Design review of the part built by this model. Coordinates are the model's own, in mm. Face numbers are marked on the shaded views. A direction names the side the tool comes from. Coordinates: 2 decimals unless noted, no trailing zeros. Order: outer loops, then holes, each group sorted by start corner. A loop starts at its lowest first (then second) coordinate and runs counter-clockwise, first axis right, second up. Notation, with made-up numbers: (61, 83.5) -> (110, 83.5) arc R26 cw to (110, 97.5) -> close; hole circle Ø11 at (52.5, 71.25). An arc over 180 degrees is marked (long way). Write item = value, one per line.
```python
from build123d import *

# Parameters (mm, degrees)
SKETCH1_W                    = 160
SKETCH1_H                    = 120
BOSS_EXTRUDE1_DEPTH          = 70
CUT_EXTRUDE1_DEPTH           = 70
M20_TAPPED_HOLE3_D           = 17.5
M20_TAPPED_HOLE3_DEPTH       = 30
M20_TAPPED_HOLE3_CBORE_D     = 20
M20_TAPPED_HOLE3_CBORE_DEPTH = 25
M20_TAPPED_HOLE3_TIP         = 5.257530416
F_20_0MM_DOWEL_SLOT1_D       = 20
F_20_0MM_DOWEL_SLOT1_DEPTH   = 40
F_20_0MM_DOWEL_SLOT1_TIP     = 6.00860619
SKETCH16_R                   = 10
CUT_EXTRUDE3_DEPTH           = 40
CUT_EXTRUDE4_DEPTH           = 40
SKETCH18_R                   = 10
BOSS_EXTRUDE2_DEPTH          = 40
CUT_EXTRUDE6_DEPTH           = 20
SKETCH20_R                   = 10
CUT_EXTRUDE7_DEPTH           = 71
SKETCH21_R                   = 10
CUT_EXTRUDE8_DEPTH           = 20
CUT_EXTRUDE11_DEPTH          = 20
CUT_EXTRUDE12_DEPTH          = 20
SKETCH25_R                   = 20
SKETCH25_R_2                 = 10
BOSS_EXTRUDE6_DEPTH          = 10
RIB1_REACH                   = 186.662
SKETCH26_WALL_W              = 391.050063724
SKETCH26_WALL_H              = 10


with BuildPart() as part:
    # Sketch1 → Boss-Extrude1 (new body)
    with BuildSketch(Plane.XY):
        with Locations((80, 60)):
            Rectangle(SKETCH1_W, SKETCH1_H)
    extrude(amount=BOSS_EXTRUDE1_DEPTH)

    # Sketch2 → Cut-Extrude1 (cut)
    with BuildSketch(Plane.XY.offset(70)):
        with BuildLine():
            Line((60, 120), (0, 120))
            Line((0, 120), (0, 60))
            ThreePointArc((0, 60), (17.573593129, 102.426406871), (60, 120))
        make_face()
        with BuildLine():
            ThreePointArc((60, 0), (17.573593129, 17.573593129), (0, 60))
            Line((0, 60), (0, 0))
            Line((0, 0), (60, 0))
        make_face()
    extrude(amount=-CUT_EXTRUDE1_DEPTH, mode=Mode.SUBTRACT)

    # M20 Tapped Hole3
    with Locations(Plane(origin=(140, 100, 70), x_dir=(1, 0, 0), z_dir=(0, 0, 1))):
        with Locations((0, 0), (0, -80)):
            CounterBoreHole(M20_TAPPED_HOLE3_D / 2, M20_TAPPED_HOLE3_CBORE_D / 2, M20_TAPPED_HOLE3_CBORE_DEPTH, depth=M20_TAPPED_HOLE3_DEPTH)
            with Locations((0, 0, -(M20_TAPPED_HOLE3_DEPTH + M20_TAPPED_HOLE3_TIP / 2))):  # 118° drill point
                Cone(0, M20_TAPPED_HOLE3_D / 2, M20_TAPPED_HOLE3_TIP, mode=Mode.SUBTRACT)

    # 20.0mm Dowel Slot1
    with Locations(Plane.XY.offset(70)):
        with Locations((60, 60)):
            Hole(F_20_0MM_DOWEL_SLOT1_D / 2, depth=F_20_0MM_DOWEL_SLOT1_DEPTH)
            with Locations((0, 0, -(F_20_0MM_DOWEL_SLOT1_DEPTH + F_20_0MM_DOWEL_SLOT1_TIP / 2))):  # 118° drill point
                Cone(0, F_20_0MM_DOWEL_SLOT1_D / 2, F_20_0MM_DOWEL_SLOT1_TIP, mode=Mode.SUBTRACT)

    # Sketch16 → Cut-Extrude3 (cut)
    with BuildSketch(Plane.XY.offset(70)):
        with BuildLine():
            ThreePointArc((28.775010008, 35), (100, 60), (28.775010008, 85))
            Line((28.775010008, 85), (5.456439427, 85))
            ThreePointArc((5.456439427, 85), (0, 60), (5.456439427, 35))
            Line((5.456439427, 35), (28.775010008, 35))
        make_face()
        with Locations((60, 60)):
            Circle(SKETCH16_R, mode=Mode.SUBTRACT)
    extrude(amount=-CUT_EXTRUDE3_DEPTH, mode=Mode.SUBTRACT)

    # Sketch17 → Cut-Extrude4 (cut)
    with BuildSketch(Plane.XY.offset(30)):
        with BuildLine():
            Line((5.456439427, 85), (28.775010008, 85))
            ThreePointArc((28.775010008, 85), (42.679491924, 96.055512755), (60, 100))
            Line((60, 100), (15.27864045, 100))
            ThreePointArc((15.27864045, 100), (9.804072956, 92.868965731), (5.456439427, 85))
        make_face()
        with BuildLine():
            Line((28.775010008, 35), (5.456439427, 35))
            ThreePointArc((5.456439427, 35), (9.804072956, 27.131034269), (15.27864045, 20))
            Line((15.27864045, 20), (60, 20))
            ThreePointArc((60, 20), (42.679491924, 23.944487245), (28.775010008, 35))
        make_face()
    extrude(amount=CUT_EXTRUDE4_DEPTH, mode=Mode.SUBTRACT)

    # Sketch18 → Boss-Extrude2 (add)
    with BuildSketch(Plane.XY.offset(30)):
        with BuildLine():
            Line((60, 20), (15.27864045, 20))
            ThreePointArc((15.27864045, 20), (0, 60), (15.27864045, 100))
            Line((15.27864045, 100), (60, 100))
            ThreePointArc((60, 100), (100, 60), (60, 20))
        make_face()
        with Locations((60, 60)):
            Circle(SKETCH18_R, mode=Mode.SUBTRACT)
    extrude(amount=BOSS_EXTRUDE2_DEPTH)

    # Sketch19 → Cut-Extrude6 (cut)
    with BuildSketch(Plane(origin=(0, 0, 0), x_dir=(-1, 0, 0), z_dir=(0, 0, -1))):
        with BuildLine():
            ThreePointArc((-60, 99.05124838), (-43.43620227, 95.364397418), (-30, 85))
            Line((-30, 85), (-5.456439427, 85))
            ThreePointArc((-5.456439427, 85), (-9.461419592, 92.339633429), (-14.447832104, 99.05124838))
            Line((-14.447832104, 99.05124838), (-60, 99.05124838))
        make_face()
        with BuildLine():
            Line((-5.456439427, 85), (-30, 85))
            ThreePointArc((-30, 85), (-43.43620227, 95.364397418), (-60, 99.05124838))
            ThreePointArc((-60, 99.05124838), (-99.05124838, 60), (-60, 20.94875162))
            ThreePointArc((-60, 20.94875162), (-43.43620227, 24.635602582), (-30, 35))
            Line((-30, 35), (-5.456439427, 35))
            ThreePointArc((-5.456439427, 35), (0, 60), (-5.456439427, 85))
        make_face()
        with BuildLine():
            ThreePointArc((-14.447832104, 20.94875162), (-9.461419592, 27.660366571), (-5.456439427, 35))
            Line((-5.456439427, 35), (-30, 35))
            ThreePointArc((-30, 35), (-43.43620227, 24.635602582), (-60, 20.94875162))
            Line((-60, 20.94875162), (-14.447832104, 20.94875162))
        make_face()
    extrude(amount=-CUT_EXTRUDE6_DEPTH, mode=Mode.SUBTRACT)

    # Sketch20 → Cut-Extrude7 (cut)
    with BuildSketch(Plane.XY.offset(70)):
        with Locations(Location((60, 60, 0), (0, 0, 180))):
            Circle(SKETCH20_R)
    extrude(amount=-CUT_EXTRUDE7_DEPTH, mode=Mode.SUBTRACT)

    # Sketch21 → Cut-Extrude8 (cut)
    with BuildSketch(Plane.XY.offset(70)):
        with BuildLine():
            Line((30, 35), (5.456439427, 35))
            ThreePointArc((5.456439427, 35), (9.461419592, 27.660366571), (14.447832104, 20.94875162))
            Line((14.447832104, 20.94875162), (60, 20.94875162))
            ThreePointArc((60, 20.94875162), (43.43620227, 24.635602582), (30, 35))
        make_face()
        with BuildLine():
            Line((5.456439427, 85), (30, 85))
            ThreePointArc((30, 85), (43.43620227, 95.364397418), (60, 99.05124838))
            Line((60, 99.05124838), (14.447832104, 99.05124838))
            ThreePointArc((14.447832104, 99.05124838), (9.461419592, 92.339633429), (5.456439427, 85))
        make_face()
        with BuildLine():
            ThreePointArc((60, 99.05124838), (43.43620227, 95.364397418), (30, 85))
            Line((30, 85), (5.456439427, 85))
            ThreePointArc((5.456439427, 85), (0, 60), (5.456439427, 35))
            Line((5.456439427, 35), (30, 35))
            ThreePointArc((30, 35), (43.43620227, 24.635602582), (60, 20.94875162))
            ThreePointArc((60, 20.94875162), (99.05124838, 60), (60, 99.05124838))
        make_face()
        with Locations(Location((60, 60, 0), (0, 0, 180))):
            Circle(SKETCH21_R, mode=Mode.SUBTRACT)
    extrude(amount=-CUT_EXTRUDE8_DEPTH, mode=Mode.SUBTRACT)

    # Sketch22 → Cut-Extrude11 (cut)
    with BuildSketch(Plane.XY.offset(50)):
        with BuildLine():
            ThreePointArc((60, 99.05124838), (43.43620227, 95.364397418), (30, 85))
            Line((30, 85), (5.456439427, 85))
            ThreePointArc((5.456439427, 85), (4.387727415, 82.522769322), (3.431457505, 80))
            Line((3.431457505, 80), (60, 80))
            ThreePointArc((60, 80), (74.142135624, 74.142135624), (80, 60))
            ThreePointArc((80, 60), (74.142135624, 45.857864376), (60, 40))
            Line((60, 40), (3.431457505, 40))
            ThreePointArc((3.431457505, 40), (4.387727415, 37.477230678), (5.456439427, 35))
            Line((5.456439427, 35), (30, 35))
            ThreePointArc((30, 35), (43.43620227, 24.635602582), (60, 20.94875162))
            ThreePointArc((60, 20.94875162), (99.05124838, 60), (60, 99.05124838))
        make_face()
    extrude(amount=-CUT_EXTRUDE11_DEPTH, mode=Mode.SUBTRACT)

    # Sketch23 → Cut-Extrude12 (cut)
    with BuildSketch(Plane.XY.offset(50)):
        with BuildLine():
            ThreePointArc((60, 40), (40, 60), (60, 80))
            Line((60, 80), (3.431457505, 80))
            ThreePointArc((3.431457505, 80), (0, 60), (3.431457505, 40))
            Line((3.431457505, 40), (60, 40))
        make_face()
    extrude(amount=-CUT_EXTRUDE12_DEPTH, mode=Mode.SUBTRACT)

    # Sketch25 → Boss-Extrude6 (add)
    with BuildSketch(Plane.XY.offset(50)):
        with Locations((60, 60)):
            Circle(SKETCH25_R)
        with Locations(Location((60, 60, 0), (0, 0, 180))):
            Circle(SKETCH25_R_2, mode=Mode.SUBTRACT)
    extrude(amount=BOSS_EXTRUDE6_DEPTH)

    # Sketch26 wall → Rib1 (add, up to next)
    with BuildSketch(Plane(origin=(89.34113782, 60, 59.598387785), x_dir=(1, 0, 0), z_dir=(0, 0, -1)), mode=Mode.PRIVATE) as rib1_sk1:
        Rectangle(SKETCH26_WALL_W, SKETCH26_WALL_H)
    rib1_tool1 = extrude(rib1_sk1.sketch, amount=RIB1_REACH, mode=Mode.PRIVATE) - part.part
    add(rib1_tool1.solids().sort_by_distance((89.34113782, 60, 59.598387785))[0])


solid = part.part
```
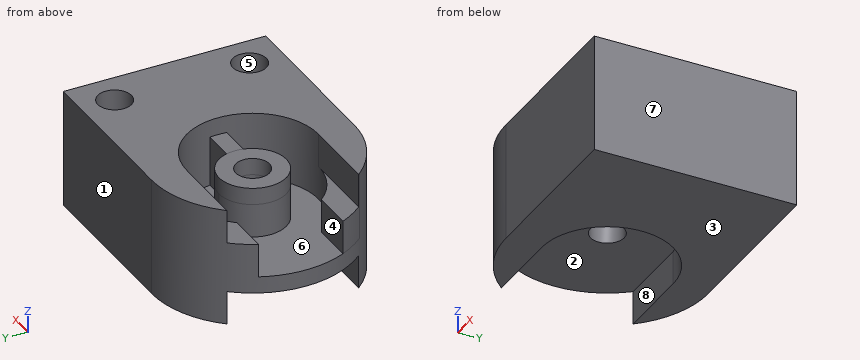
(1) Insertion check: pin 1 (10 mm diameter, centred on x = 139.5, y = 19, fed in from +Z); pin 2 (1.5 mm diameter, centred on x = 28, y = 49.5, fed in from -Z); pin 3 (4 mm diameter, centred on x = 43, y = 92.5, fed in from +Z); pin 4 (12 mm diameter, centred on x = 60, y = 60, fed in from +Z). Each pin has a flat end and moves straight along its axis. Give the tip position at first contact, or say it passes through.
Report:
pin_1 = 38.42
pin_2 = 20
pin_3 = 30
pin_4 = through
(2) We need section C-C (x = 96). Write out the cut boundary in (y, z).
Report:
outline = (0, 0) -> (44.87, 0) -> (44.87, 20) -> (75.13, 20) -> (75.13, 0) -> (120, 0) -> (120, 70) -> (75.13, 70) -> (75.13, 30) -> (65, 30) -> (65, 59.6) -> (55, 59.6) -> (55, 30) -> (44.87, 30) -> (44.87, 70) -> (0, 70) -> close
(3) For L1, parallel to Y at x = 140, z = 43; L2, parallel to Y at x = 140, z = 65; L3, parallel to X at y = 60, z = 57, list the stretches that pass through material, from the lowest coordinate up.
Report:
L1 = 0 to 11.25, 28.75 to 91.25, 108.75 to 120
L2 = 0 to 10, 30 to 90, 110 to 120
L3 = 40 to 50, 70 to 160
(4) The part is to be moulded in two halves that separate along X. For the marked faces 6, 7 and 8, say which applies: released by +X, released by -X, zero draft, split by the parting line, or undercut.
Report:
face_6 = undercut
face_7 = released by +X
face_8 = zero draft
(5) We need section B-B (x = 56). Write out the cut boundary in (y, z), and give its area (3 significant figures).
Report:
outline = (0.13, 0) -> (20.95, 0) -> (20.95, 20) -> (50.83, 20) -> (50.83, 60) -> (40.4, 60) -> (40.4, 30) -> (21.15, 30) -> (21.15, 50) -> (20.95, 50) -> (20.95, 70) -> (0.13, 70) -> close; (69.17, 20) -> (99.05, 20) -> (99.05, 0) -> (119.87, 0) -> (119.87, 70) -> (99.05, 70) -> (99.05, 50) -> (98.85, 50) -> (98.85, 30) -> (79.6, 30) -> (79.6, 60) -> (69.17, 60) -> close
area = 4,150 mm²
(6) We need section A-A (y = 52.5). Write out the cut boundary in (x, z), and give its area (3 significant figures).
Report:
outline = (0.47, 20) -> (53.39, 20) -> (53.39, 60) -> (41.46, 60) -> (41.46, 30) -> (0.47, 30) -> close; (66.61, 20) -> (98.32, 20) -> (98.32, 0) -> (160, 0) -> (160, 70) -> (98.32, 70) -> (98.32, 30) -> (78.54, 30) -> (78.54, 60) -> (66.61, 60) -> close
area = 5,880 mm²
(7) For the marked faces 1, 2, 3, 4 and 5, list the 3-axis set-ups (+Z, -Z, +X, -X, +Y, -Y) from which the entire face can be reached by the end or side of a thin tool; tool diameter is ignored.
Report:
face_1 = +Z, -Z, +X, -X, +Y
face_2 = -Z, -X
face_3 = -Z, +X, -X, +Y, -Y
face_4 = +Z, -X
face_5 = +Z
